```python
from build123d import *

# Parameters (mm, degrees)
SKETCH1_R           = 1
SKETCH1_R_2         = 1.616439125
BOSS_EXTRUDE4_DEPTH = 0.381


with BuildPart() as part:
    # Sketch1 → Boss-Extrude4 (new body)
    with BuildSketch(Plane(origin=(0, 0, 0), x_dir=(1, 0, 0), z_dir=(0, 1, 0))):
        with BuildLine():
            Line((4.461504525, -1.55), (10, -1.55))
            Line((10, -1.55), (10, -2))
            ThreePointArc((10, -2), (10.292893219, -2.707106781), (11, -3))
            Line((11, -3), (14.538495475, -3))
            ThreePointArc((14.538495475, -3), (15.245602257, -2.707106781), (15.538495475, -2))
            Line((15.538495475, -2), (15.538495475, 2))
            ThreePointArc((15.538495475, 2), (15.245602257, 2.707106781), (14.538495475, 3))
            Line((14.538495475, 3), (11, 3))
            ThreePointArc((11, 3), (10.292893219, 2.707106781), (10, 2))
            Line((10, 2), (10, 1.55))
            Line((10, 1.55), (4.461504525, 1.55))
            ThreePointArc((4.461504525, 1.55), (0, 0), (4.461504525, -1.55))
        make_face()
        with Locations((2.5, 0)):
            Circle(SKETCH1_R, mode=Mode.SUBTRACT)
        with Locations((13.839657546, 0)):
            Circle(SKETCH1_R_2, mode=Mode.SUBTRACT)
    extrude(amount=BOSS_EXTRUDE4_DEPTH)


solid = part.part
```
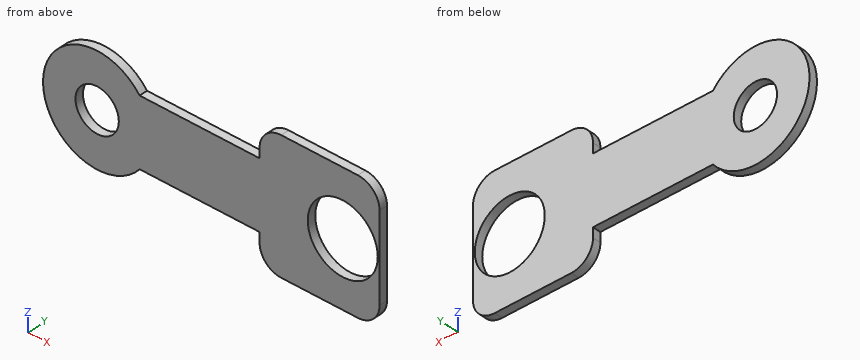
Build history of the part. All positions in model axes, mm. Round coordinates to 2 decimals unless told otherwise and drop trailing zeros. Loops run counter-clockwise (first coordinate to the right, second up) from the corner with the lowest first, then second, coordinate; pieces in that order, holes last. Notation, with made-up numbers: M 4.25,-23 L 25.25,-23 A19 cw 25.25,2 Z; hole C 15.5,-6.75 d4. An arc over 180 degrees is marked long. Answer as CSV lines item,"result".
1. Flat gauge pin, fed straight in: P1, Ø1.8, axis at x = 2.5, z = 0, coming from the -Y side. Where does the tip first touch, or does it go through?
Resolved:
P1,"passes through"
2. Cut at D-D on x = 12.75. Write the cut outline in (y, z).
Resolved:
outline,"M 0,-3 L 0.38,-3 L 0.38,-1.19 L 0,-1.19 Z; M 0,1.19 L 0.38,1.19 L 0.38,3 L 0,3 Z"
3. Cut at B-B on x = 2.5. Write the cut outline in (y, z), then the cut area to 3 significant figures.
Resolved:
outline,"M 0,-2.5 L 0.38,-2.5 L 0.38,-1 L 0,-1 Z; M 0,1 L 0.38,1 L 0.38,2.5 L 0,2.5 Z"
area,"1.14 mm²"
4. Cut at C-C on y = 0.3. Write the cut outline in (x, z).
Resolved:
outline,"M 4.46,-1.55 L 10,-1.55 L 10,-2 A1 ccw 11,-3 L 14.54,-3 A1 ccw 15.54,-2 L 15.54,2 A1 ccw 14.54,3 L 11,3 A1 ccw 10,2 L 10,1.55 L 4.46,1.55 A2.5 ccw long Z; hole C 2.5,0 d2; hole C 13.84,0 d3.23"
5. Wall check: probe 1 along Z at (x, y) = (2.5, 0.1); probe 2 along Z at (x, y) = (6.75, 0.1); probe 3 along Z at (x, y) = (14.25, 0.25). Give the ranges that are in metal, low to high. Write a range as [from, to].
Resolved:
probe 1,"z = [-2.5, -1], [1, 2.5]"
probe 2,"z = [-1.55, 1.55]"
probe 3,"z = [-3, -1.56], [1.56, 3]"
6. Cut at A-A on z = 0. Write the cut outline in (x, y).
Resolved:
outline,"M 0,0 L 1.5,0 L 1.5,0.38 L 0,0.38 Z; M 3.5,0 L 12.22,0 L 12.22,0.38 L 3.5,0.38 Z; M 15.46,0 L 15.54,0 L 15.54,0.38 L 15.46,0.38 Z"
